Design review of the part built by this model. Coordinates are the model's own, in mm. A direction names the side the tool comes from. Give positions to 0.01 mm unless a question says otherwise; leave off trailing zeros. Loops run counter-clockwise (first coordinate to the right, second up) from the corner with the lowest first, then second, coordinate; pieces in that order, holes last.
from build123d import *

# Parameters (mm, degrees)
SKETCH1_W           = 43
SKETCH1_H           = 21
BOSS_EXTRUDE1_DEPTH = 2
SKETCH2_W           = 41.4
SKETCH2_H           = 19.4
SKETCH2_W_2         = 39.6
SKETCH2_H_2         = 17.6
BOSS_EXTRUDE2_DEPTH = 1.8
CUT_EXTRUDE1_DEPTH  = 25.010414407
FILL_PATTERN1_DEPTH = 2
SKETCH4_W           = 21.566848352
SKETCH4_H           = 13.5
CUT_EXTRUDE4_DEPTH  = 25.226844615


# Read off the part's stored shape, not the designer's step: Fill Pattern1
with BuildPart() as part:
    # Sketch1 → Boss-Extrude1 (new body)
    with BuildSketch(Plane.XY):
        Rectangle(SKETCH1_W, SKETCH1_H)
    extrude(amount=BOSS_EXTRUDE1_DEPTH)

    # Sketch2 → Boss-Extrude2 (add)
    with BuildSketch(Plane.XY.offset(2)):
        Rectangle(SKETCH2_W, SKETCH2_H)
        Rectangle(SKETCH2_W_2, SKETCH2_H_2, mode=Mode.SUBTRACT)
    extrude(amount=BOSS_EXTRUDE2_DEPTH)

    # Sketch3 → Cut-Extrude1 (cut, through all)
    with BuildSketch(Plane.XY.offset(2)):
        Polygon((-0.866025404, 1.5), (-1.732050808, 0), (-0.866025404, -1.5), (0.866025404, -1.5), (1.732050808, 0), (0.866025404, 1.5), align=None)
    extrude(amount=-CUT_EXTRUDE1_DEPTH, mode=Mode.SUBTRACT)

    # Fill Pattern1 outline → Fill Pattern1 (cut)
    with BuildSketch(Plane.XY):
        Polygon((7.794228634, 0), (6.92820323, 1.5), (5.196152423, 1.5), (4.330127019, 0), (5.196152423, -1.5), (6.92820323, -1.5), align=None)
        Polygon((13.856406461, 0), (12.990381057, 1.5), (11.258330249, 1.5), (10.392304845, 0), (11.258330249, -1.5), (12.990381057, -1.5), align=None)
        Polygon((-4.330127019, 0), (-5.196152423, 1.5), (-6.92820323, 1.5), (-7.794228634, 0), (-6.92820323, -1.5), (-5.196152423, -1.5), align=None)
        Polygon((-10.392304845, 0), (-11.258330249, 1.5), (-12.990381057, 1.5), (-13.856406461, 0), (-12.990381057, -1.5), (-11.258330249, -1.5), align=None)
        Polygon((-2.165063509, 3.75), (-1.299038106, 5.25), (-2.165063509, 6.75), (-3.897114317, 6.75), (-4.763139721, 5.25), (-3.897114317, 3.75), align=None)
        Polygon((3.897114317, -6.75), (4.763139721, -5.25), (3.897114317, -3.75), (2.165063509, -3.75), (1.299038106, -5.25), (2.165063509, -6.75), align=None)
        Polygon((-3.897114317, -6.75), (-2.165063509, -6.75), (-1.299038106, -5.25), (-2.165063509, -3.75), (-3.897114317, -3.75), (-4.763139721, -5.25), align=None)
        Polygon((2.165063509, 3.75), (3.897114317, 3.75), (4.763139721, 5.25), (3.897114317, 6.75), (2.165063509, 6.75), (1.299038106, 5.25), align=None)
        Polygon((16.887495374, -5.25), (16.02146997, -3.75), (14.289419162, -3.75), (13.423393759, -5.25), (14.289419162, -6.75), (16.02146997, -6.75), align=None)
        Polygon((-7.361215932, -5.25), (-8.227241336, -3.75), (-9.959292144, -3.75), (-10.825317547, -5.25), (-9.959292144, -6.75), (-8.227241336, -6.75), align=None)
        Polygon((10.825317547, -5.25), (9.959292144, -3.75), (8.227241336, -3.75), (7.361215932, -5.25), (8.227241336, -6.75), (9.959292144, -6.75), align=None)
        Polygon((-13.423393759, -5.25), (-14.289419162, -3.75), (-16.02146997, -3.75), (-16.887495374, -5.25), (-16.02146997, -6.75), (-14.289419162, -6.75), align=None)
        Polygon((9.959292144, 3.75), (10.825317547, 5.25), (9.959292144, 6.75), (8.227241336, 6.75), (7.361215932, 5.25), (8.227241336, 3.75), align=None)
        Polygon((-10.392304845, 3.5), (-11.258330249, 5), (-12.990381057, 5), (-13.856406461, 3.5), (-12.990381057, 2), (-11.258330249, 2), align=None)
        Polygon((13.856406461, 3.5), (12.990381057, 5), (11.258330249, 5), (10.392304845, 3.5), (11.258330249, 2), (12.990381057, 2), align=None)
        Polygon((1.732050808, 3.5), (0.866025404, 5), (-0.866025404, 5), (-1.732050808, 3.5), (-0.866025404, 2), (0.866025404, 2), align=None)
        Polygon((-4.330127019, 3.5), (-5.196152423, 5), (-6.92820323, 5), (-7.794228634, 3.5), (-6.92820323, 2), (-5.196152423, 2), align=None)
        Polygon((7.794228634, 3.5), (6.92820323, 5), (5.196152423, 5), (4.330127019, 3.5), (5.196152423, 2), (6.92820323, 2), align=None)
        Polygon((-8.227241336, -3.25), (-7.361215932, -1.75), (-8.227241336, -0.25), (-9.959292144, -0.25), (-10.825317547, -1.75), (-9.959292144, -3.25), align=None)
        Polygon((-16.02146997, -3.25), (-14.289419162, -3.25), (-13.423393759, -1.75), (-14.289419162, -0.25), (-16.02146997, -0.25), (-16.887495374, -1.75), align=None)
        Polygon((-7.361215932, 5.25), (-8.227241336, 6.75), (-9.959292144, 6.75), (-10.825317547, 5.25), (-9.959292144, 3.75), (-8.227241336, 3.75), align=None)
        Polygon((-13.423393759, 5.25), (-14.289419162, 6.75), (-16.02146997, 6.75), (-16.887495374, 5.25), (-16.02146997, 3.75), (-14.289419162, 3.75), align=None)
        Polygon((16.887495374, 5.25), (16.02146997, 6.75), (14.289419162, 6.75), (13.423393759, 5.25), (14.289419162, 3.75), (16.02146997, 3.75), align=None)
        Polygon((-13.423393759, 1.75), (-14.289419162, 3.25), (-16.02146997, 3.25), (-16.887495374, 1.75), (-16.02146997, 0.25), (-14.289419162, 0.25), align=None)
        Polygon((10.825317547, 1.75), (9.959292144, 3.25), (8.227241336, 3.25), (7.361215932, 1.75), (8.227241336, 0.25), (9.959292144, 0.25), align=None)
        Polygon((16.887495374, 1.75), (16.02146997, 3.25), (14.289419162, 3.25), (13.423393759, 1.75), (14.289419162, 0.25), (16.02146997, 0.25), align=None)
        Polygon((-1.299038106, 1.75), (-2.165063509, 3.25), (-3.897114317, 3.25), (-4.763139721, 1.75), (-3.897114317, 0.25), (-2.165063509, 0.25), align=None)
        Polygon((-7.361215932, 1.75), (-8.227241336, 3.25), (-9.959292144, 3.25), (-10.825317547, 1.75), (-9.959292144, 0.25), (-8.227241336, 0.25), align=None)
        Polygon((4.763139721, 1.75), (3.897114317, 3.25), (2.165063509, 3.25), (1.299038106, 1.75), (2.165063509, 0.25), (3.897114317, 0.25), align=None)
        Polygon((-11.258330249, -5), (-10.392304845, -3.5), (-11.258330249, -2), (-12.990381057, -2), (-13.856406461, -3.5), (-12.990381057, -5), align=None)
        Polygon((4.763139721, -1.75), (3.897114317, -0.25), (2.165063509, -0.25), (1.299038106, -1.75), (2.165063509, -3.25), (3.897114317, -3.25), align=None)
        Polygon((16.887495374, -1.75), (16.02146997, -0.25), (14.289419162, -0.25), (13.423393759, -1.75), (14.289419162, -3.25), (16.02146997, -3.25), align=None)
        Polygon((10.825317547, -1.75), (9.959292144, -0.25), (8.227241336, -0.25), (7.361215932, -1.75), (8.227241336, -3.25), (9.959292144, -3.25), align=None)
        Polygon((-1.299038106, -1.75), (-2.165063509, -0.25), (-3.897114317, -0.25), (-4.763139721, -1.75), (-3.897114317, -3.25), (-2.165063509, -3.25), align=None)
        Polygon((1.732050808, -3.5), (0.866025404, -2), (-0.866025404, -2), (-1.732050808, -3.5), (-0.866025404, -5), (0.866025404, -5), align=None)
        Polygon((13.856406461, -3.5), (12.990381057, -2), (11.258330249, -2), (10.392304845, -3.5), (11.258330249, -5), (12.990381057, -5), align=None)
        Polygon((7.794228634, -3.5), (6.92820323, -2), (5.196152423, -2), (4.330127019, -3.5), (5.196152423, -5), (6.92820323, -5), align=None)
        Polygon((-4.330127019, -3.5), (-5.196152423, -2), (-6.92820323, -2), (-7.794228634, -3.5), (-6.92820323, -5), (-5.196152423, -5), align=None)
    extrude(amount=FILL_PATTERN1_DEPTH, mode=Mode.SUBTRACT)

    # Sketch4 → Cut-Extrude4 (cut, through all)
    with BuildSketch(Plane(origin=(0, 0, 0), x_dir=(-1, 0, 0), z_dir=(0, 0, -1))):
        with Locations((6.886309859, 0)):
            Rectangle(SKETCH4_W, SKETCH4_H)
    extrude(amount=-CUT_EXTRUDE4_DEPTH, mode=Mode.SUBTRACT)


solid = part.part
Q1. Tool access review of faces 1 (the face through (4.336, 5.99, 0.986)), 2 (the face through (0, -10.5, 1)), 3 (the face through (0, -8.8, 3)): name each direction out of +Z, -Z, +X, -X, +Y, -Y from which nothing blocks a thin tool from reaching the whole face with its end or side.
Results:
face 1: +Z, -Z
face 2: +Z, -Z, +X, -X, -Y
face 3: +Z
Q2. Take a section at C-C (z = 3.2). Give the boundary of the cut face in (x, y), plus the area to 3 significant figures.
Results:
outline: (-20.7, -9.7) - (20.7, -9.7) - (20.7, 9.7) - (-20.7, 9.7) - close; hole (-19.8, -8.8) - (19.8, -8.8) - (19.8, 8.8) - (-19.8, 8.8) - close
area: 106 mm2
Q3. Take a section at B-B (x = 0.5). Give the boundary of the cut face in (y, z).
Results:
outline: (-10.5, 0) - (-6.75, 0) - (-6.75, 2) - (-8.8, 2) - (-8.8, 3.8) - (-9.7, 3.8) - (-9.7, 2) - (-10.5, 2) - close; (6.75, 0) - (10.5, 0) - (10.5, 2) - (9.7, 2) - (9.7, 3.8) - (8.8, 3.8) - (8.8, 2) - (6.75, 2) - close
Q4. Draft analysis for pull direction X (two halves, no side actions). For faces 4 (the face through (20.7, 0, 3)), 5 (the face through (-17.67, 0, 1)), 6 (the face through (13.86, -0.99, 0.99)), 7 (the face through (-6, -10, 2)), state which applies: pulls with the +X half, pulls with the -X half, needs draft (parallel to the pull), parting line crosses it, or undercut.
Results:
face 4: pulls with the +X half
face 5: undercut
face 6: undercut
face 7: needs draft
Q5. Insertion check: pin 1 (5 mm diameter, centred on x = 5, y = 2.5, fed in from +Z). The pin has a flat end and moves straight along its axis. Give the tip position at first contact, or say it passes through.
Results:
pin 1: stops at z = 2
Q6. Take a section at A-A (x = 9.5). Give the boundary of the cut face in (y, z).
Results:
outline: (-10.5, 0) - (-6.75, 0) - (-6.75, 2) - (-8.8, 2) - (-8.8, 3.8) - (-9.7, 3.8) - (-9.7, 2) - (-10.5, 2) - close; (-3.75, 0) - (-3.25, 0) - (-3.25, 2) - (-3.75, 2) - close; (-0.25, 0) - (0.25, 0) - (0.25, 2) - (-0.25, 2) - close; (3.25, 0) - (3.75, 0) - (3.75, 2) - (3.25, 2) - close; (6.75, 0) - (10.5, 0) - (10.5, 2) - (9.7, 2) - (9.7, 3.8) - (8.8, 3.8) - (8.8, 2) - (6.75, 2) - close
Q7. Take a section at D-D (y = -4.25). Give the number of separate pieces and of enclosed holes in the cut face, plus the area to 3 significant figures.
Results:
separate pieces: 6
enclosed holes: 0
area: 25.9 mm2
Q8. Wall thickness on line 1 (Y direction, x = 6, z = 0.6); line 2 (X direction, y = -1.75, z = 1.3); line 3 (Y direction, x = -1, z = 2.9): over which ranges is each line inside the solid? List them lowest first.
Results:
line 1: y = -10.5 to -5, -2 to -1.5, 1.5 to 2, 5 to 10.5
line 2: x = -21.5 to -17.67, 4.76 to 7.36, 10.83 to 13.42, 16.89 to 21.5
line 3: y = -9.7 to -8.8, 8.8 to 9.7
